Verification items for the finished model (mm, model axes). Face numbers are marked on the shaded views. A direction names the side the tool comes from. Round coordinates to 2 decimals unless told otherwise and drop trailing zeros. Loops run counter-clockwise (first coordinate to the right, second up) from the corner with the lowest first, then second, coordinate; pieces in that order, holes last. Notation, with made-up numbers: (54, 24.25) -> (63, 24.25) arc R33 cw to (63, 55.25) -> close; hole circle Ø10 at (87.5, 65.25). An arc over 180 degrees is marked (long way). Use a Markdown table: item, result. Add a question column.
```python
from build123d import *

# Parameters (mm, degrees)
F0_R     = 22.5
F1_DEPTH = 20


# Not quite as in the source:
# - a feature names something its author has since deleted; it is built from what else it names


with BuildPart() as f1:
    # F0 (on Front) → F1 (new body)
    with BuildSketch(Plane.XZ):
        Polygon((37.5, 50), (-40, 50), (-50, 50), (-50, 40), (-50, -40), (-50, -41.9841893017), (-50, -50), (-40, -50), (-25, -50), (0, -50), (25, -50), (40, -50), (50, -50), (50, -41.9841893017), (50, -40), (50, 40), (50, 50), (40, 50), align=None)
        Circle(F0_R, mode=Mode.SUBTRACT)
        with BuildLine():
            ThreePointArc((-25, -50), (-22.6149008919, -63.790810636), (-32.2747059634, -73.9181657563))
            ThreePointArc((-32.2747059634, -73.9181657563), (-10.1149008919, -70.0856621634), (0, -50))
            Line((0, -50), (-25, -50))
        make_face()
        with BuildLine():
            Line((25, -50), (0, -50))
            ThreePointArc((0, -50), (10.1268327857, -70.0944991731), (32.3031117614, -73.909507703))
            ThreePointArc((32.3031117614, -73.909507703), (22.6268327857, -63.7949935854), (25, -50))
        make_face()
    extrude(amount=F1_DEPTH)


solid = f1.part
```
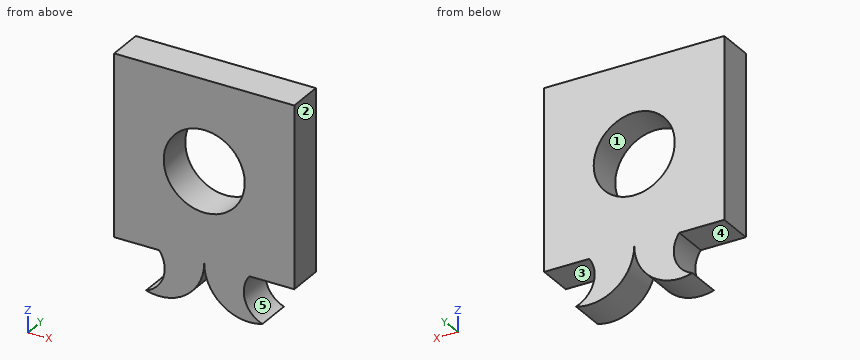
1) Sectioned sample at D-D on x = -35. Enter the section's corners in (y, z), then the cut area to 3 significant figures.
2) Release check for a two-part mould opening along X. For the marked faces 1, 2 and 3 record: released by +X, released by -X, zero draft, split by the parting line, or undercut.
3) Sectioned sample at A-A on z = 0. Enter the section's corners in (x, y), then the cut area to 3 significant figures.
4) Thickness scan on line 1 (Z direction, x = 3.5, y = -5.5); line 2 (Z direction, x = 11, y = -4.5); line 3 (Z direction, x = 42, y = -2.75). Record the ranges inside material, lowest first.
5) Sectioned sample at B-B on x = -15. Enter the section's corners in (y, z), then the cut area to 3 significant figures.
6) Sectioned sample at C-C on y = -2.5. Enter the section's corners in (x, z).
7) Go/stop test with a flat-tipped pin: pin 1 (10 mm diameter, centred on x = 42.5, y = -6, fed in from -Z). Record where the tip stops, or that it passes through.
8) Access from +Z, -Z, +X, -X, +Y, -Y to the whole of each face (thin tool, end or side, straight path). Record for the marked faces 4 and 5.
Geometry results:
| question | item | result |
|---|---|---|
| 1 | outline | (-20, -50) -> (0, -50) -> (0, 50) -> (-20, 50) -> close |
| 1 | area | 2,000 mm^2 |
| 2 | face 1 | undercut |
| 2 | face 2 | released by +X |
| 2 | face 3 | zero draft |
| 3 | outline | (-50, -20) -> (-22.5, -20) -> (-22.5, 0) -> (-50, 0) -> close; (22.5, -20) -> (50, -20) -> (50, 0) -> (22.5, 0) -> close |
| 3 | area | 1,100 mm^2 |
| 4 | line 1 | -62.76 to -22.23, 22.23 to 50 |
| 4 | line 2 | -70.71 to -19.63, 19.63 to 50 |
| 4 | line 3 | -50 to 50 |
| 5 | outline | (-20, -72.91) -> (0, -72.91) -> (0, -16.77) -> (-20, -16.77) -> close; (-20, 16.77) -> (0, 16.77) -> (0, 50) -> (-20, 50) -> close |
| 5 | area | 1,790 mm^2 |
| 6 | outline | (-50, -50) -> (-25, -50) arc R15.56 cw to (-32.27, -73.92) arc R25 ccw to (0, -50) arc R25 ccw to (32.3, -73.91) arc R15.55 cw to (25, -50) -> (50, -50) -> (50, 50) -> (-50, 50) -> close; hole circle Ø45 at (0, 0) |
| 7 | pin 1 | z = -50 |
| 8 | face 4 | -X, +Y, -Y |
| 8 | face 5 | +X, +Y, -Y |
